from build123d import *

# Parameters (mm, degrees)
SKETCH_1_W      = 33
SKETCH_1_H      = 43.435
EXTRUDE_1_DEPTH = 4


with BuildPart() as part:
    # 草图1 → 凸台-拉伸1 (new body)
    with BuildSketch(Plane(origin=(0, 0, 0), x_dir=(1, 0, 0), z_dir=(0, 1, 0))):
        Polygon((0, 0), (0, 95.33), (4, 96.87), (4, 2), (74, 2), (74, 96.87), (78, 95.33), (78, -95.33), (74, -96.87), (74, -49.435), (4, -49.435), (4, -96.87), (0, -95.33), align=None)
        with Locations((20.5, -23.7175)):
            Rectangle(SKETCH_1_W, SKETCH_1_H, mode=Mode.SUBTRACT)
        with Locations((57.5, -23.7175)):
            Rectangle(SKETCH_1_W, SKETCH_1_H, mode=Mode.SUBTRACT)
    extrude(amount=EXTRUDE_1_DEPTH)


solid = part.part
Read the model definition and answer for the solid it produces. Units are mm, in the model's axes. A direction names the side the tool comes from. Round coordinates to 2 decimals unless told otherwise and drop trailing zeros. Write each loop counter-clockwise with the first axis right and the second up, starting at its lowest first coordinate (ties: lowest second). Pieces come first, ordered by that corner, then holes. Notation, with made-up numbers: (-34, 15.5) - (-22, 15.5) arc R15 cw to (-22, 20.5) - close; hole circle Ø2 at (-21, 88.5). An arc over 180 degrees is marked (long way). Use a Markdown table: item, result.
(1) The part is cut by section D-D (x = 57). Write down the section's boundary in (y, z) (3 decimals).
Reported:
| item | result |
|---|---|
| outline | (0, -2) - (4, -2) - (4, 2) - (0, 2) - close; (0, 45.435) - (4, 45.435) - (4, 49.435) - (0, 49.435) - close |
(2) Straight lines are drawn through the part: line 1 along X through (y, z) = (1.4, 12); line 2 along Z through (x, y) = (65.5, 1.5) (3 decimals); line 3 along X through (y, z) = (2.65, -18). For each, find the intervals that lie inside material, in ascending order. Write a range as [from, to].
Reported:
| item | result |
|---|---|
| line 1 | [0, 4], [37, 41], [74, 78] |
| line 2 | [-2, 2], [45.435, 49.435] |
| line 3 | [0, 4], [74, 78] |
(3) Which of the six approach directions +Z, -Z, +X, -X, +Y, -Y give full straight-line access (tool end or side, diameter ignored) to faces 5 (the flat face through (74, 2, -49)), 6 (the flat face through (74, 2, 73)), 7 (the flat face through (20, 2, 45.435))?
Reported:
| item | result |
|---|---|
| face 5 | -Z, +Y, -Y |
| face 6 | +Z, +Y, -Y |
| face 7 | +Y, -Y |
(4) Each of these flat-tipped pins is pushed along its axis until it touches: pin 1 Ø1.2 at (x, y) = (25, 2.5) entering from -Z; pin 2 Ø1 at (x, y) = (70, 2.5) entering from +Z (3 decimals); pin 3 Ø4 at (x, z) = (68, 4.5) entering from +Y. Where does it stop, or does it pass through?
Reported:
| item | result |
|---|---|
| pin 1 | z = -2 |
| pin 2 | z = 49.435 |
| pin 3 | through |
(5) The mould has two halves that part along X. Classify faces 1 (the flat face through (2, 2, -96.1)), 2 (the flat face through (78, 2, -1)), 3 (the flat face through (37, 2, 24)), 4 (the flat face through (39, 0, 0)): released by +X, released by -X, zero draft, split by the parting line, or undercut.
Reported:
| item | result |
|---|---|
| face 1 | released by -X |
| face 2 | released by +X |
| face 3 | undercut |
| face 4 | zero draft |
(6) The part is cut by section B-B (z = -79.5). Write down the section's boundary in (x, y), then the cut area to 3 significant figures.
Reported:
| item | result |
|---|---|
| outline | (0, 0) - (4, 0) - (4, 4) - (0, 4) - close; (74, 0) - (78, 0) - (78, 4) - (74, 4) - close |
| area | 32.0 mm2 |
(7) The part is cut by section A-A (z = 7). Write down the section's boundary in (x, y), then the cut area to 3 significant figures.
Reported:
| item | result |
|---|---|
| outline | (0, 0) - (4, 0) - (4, 4) - (0, 4) - close; (37, 0) - (41, 0) - (41, 4) - (37, 4) - close; (74, 0) - (78, 0) - (78, 4) - (74, 4) - close |
| area | 48.0 mm2 |
(8) The part is cut by section C-C (y = 2.4). Write down the section's boundary in (x, z) (3 decimals), then the cut area to 3 significant figures.
Reported:
| item | result |
|---|---|
| outline | (0, -95.33) - (4, -96.87) - (4, -2) - (74, -2) - (74, -96.87) - (78, -95.33) - (78, 95.33) - (74, 96.87) - (74, 49.435) - (4, 49.435) - (4, 96.87) - (0, 95.33) - close; hole (4, 2) - (37, 2) - (37, 45.435) - (4, 45.435) - close; hole (41, 2) - (74, 2) - (74, 45.435) - (41, 45.435) - close |
| area | 2,270 mm2 |
